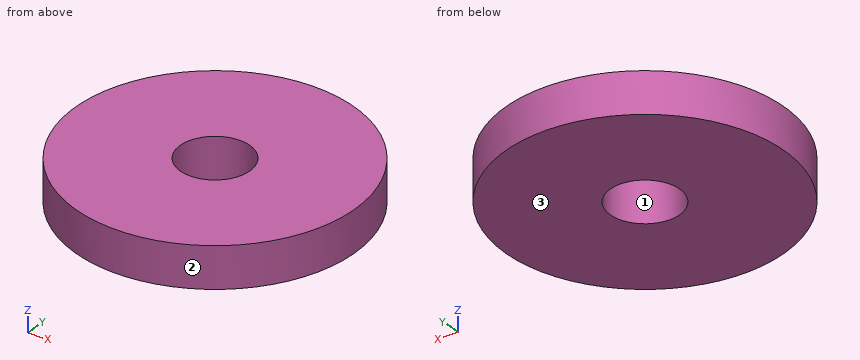
from build123d import *

# Parameters (mm, degrees)
SKETCH_1_R          = 150
EXTRUDE_1_DEPTH     = 29.535936744
SKETCH_2_R          = 25
CUT_EXTRUDE_2_DEPTH = 29.535936744
CUT_EXTRUDE_START   = -29.535936744
SKETCH_3_R          = 150
SKETCH_3_R_2        = 100
CUT_EXTRUDE_3_DEPTH = 29.535936744


with BuildPart() as part:
    # 草图1 → 凸台-拉伸1 (new body)
    with BuildSketch(Plane.XY):
        Circle(SKETCH_1_R)
    extrude(amount=EXTRUDE_1_DEPTH)

    # 草图2 → 切除-拉伸2 (cut)
    with BuildSketch(Plane.XY.offset(29.535936744)):
        Circle(SKETCH_2_R)
    extrude(amount=-CUT_EXTRUDE_2_DEPTH, mode=Mode.SUBTRACT)

    # 草图3 → 切除-拉伸3 (cut)
    with BuildSketch(Plane.XY.offset(29.535936744).offset(CUT_EXTRUDE_START)):
        Circle(SKETCH_3_R)
        Circle(SKETCH_3_R_2, mode=Mode.SUBTRACT)
    extrude(amount=CUT_EXTRUDE_3_DEPTH, mode=Mode.SUBTRACT)


solid = part.part
For this review, take the finished solid that the model builds, in its own axes (mm). Face numbers are marked on the shaded views. Give positions to 0.01 mm unless a question says otherwise; leave off trailing zeros. Order: outer loops, then holes, each group sorted by start corner. A loop starts at its lowest first (then second) coordinate and runs counter-clockwise, first axis right, second up. Notation, with made-up numbers: M -23.5,-5.75 L 7.5,-5.75 A12 ccw 7.5,7.25 Z; hole C 86,57.5 d4. An arc over 180 degrees is marked long. Answer in a Markdown table with one row per item. Add a question column.
(1) For pin 1 (10 mm diameter, centred on x = 63.5, z = 10, fed in from -Y); pin 2 (1 mm diameter, centred on y = -9.5, z = 17.5, fed in from -X); pin 3 (3 mm diameter, centred on y = 28.5, z = 15.5, fed in from -X); pin 4 (12 mm diameter, centred on y = 3, z = 8, fed in from +X), all flat-tipped, find the tip position at first contact; note any pin that passes through.
(2) Consider section D-D on x = 63. State the section outline as (y, z) points.
(3) Consider section C-C on z = 19.75. State the section outline as (x, y) points.
(4) Mouldability with a two-part tool opening along Y and no side actions: class the marked faces 1, 2 and 3 as +Y half, -Y half, draft (parallel to the pull), parting line (faces both ways), or undercut.
(5) Wall thickness on probe 1 along Y at (x, z) = (0, 13); probe 2 along X at (y, z) = (-12.5, 12); probe 3 along X at (y, z) = (15, 7): over which ranges is each line inside the solid? List them lowest first. Write a range as [from, to].
(6) Consider section A-A on y = 0. State the section outline as (x, z) points.
Evaluation:
| question | item | result |
|---|---|---|
| 1 | pin 1 | stops at y = -81.1 |
| 1 | pin 2 | stops at x = -99.59 |
| 1 | pin 3 | stops at x = -96.29 |
| 1 | pin 4 | stops at x = 100 |
| 2 | outline | M -77.66,0 L 77.66,0 L 77.66,29.54 L -77.66,29.54 Z |
| 3 | outline | C 0,0 d200; hole C 0,0 d50 |
| 4 | face 1 | undercut |
| 4 | face 2 | parting line |
| 4 | face 3 | draft |
| 5 | probe 1 | y = [-100, -25], [25, 100] |
| 5 | probe 2 | x = [-99.22, -21.65], [21.65, 99.22] |
| 5 | probe 3 | x = [-98.87, -20], [20, 98.87] |
| 6 | outline | M -100,0 L -25,0 L -25,29.54 L -100,29.54 Z; M 25,0 L 100,0 L 100,29.54 L 25,29.54 Z |
